Build history of the part. All positions in model axes, mm. Give positions to 0.01 mm unless a question says otherwise; leave off trailing zeros. Write each loop counter-clockwise with the first axis right and the second up, starting at its lowest first coordinate (ties: lowest second). Pieces come first, ordered by that corner, then holes. Notation, with made-up numbers: (52, 79.5) -> (70, 79.5) arc R37 ccw to (70, 115.5) -> close; hole circle Ø8 at (8, 16). An arc over 180 degrees is marked (long way). One line per question, with ' | ' between items. Start each with the question number.
(1) Pin check, flat tip, straight feed: P1, Ø5, axis at x = 30.75, y = -30.2, coming from the -Z side. Stop position of the tip, or through.
(2) Band-saw the part on B-B, the plane x = 0. Give the cut face in (y, z) (3 decimals).
(3) Drill centre lines: probe 1 along Y at (x, z) = (0, 19.5) (3 decimals); probe 2 along Y at (x, z) = (32, 5); probe 3 along X at (y, z) = (2, 11.75). Where is each one in solid material? Low to high. Write a range as from..to.
(4) Band-saw the part on A-A, the plane y = 0. Give the cut face in (x, z) (3 decimals).
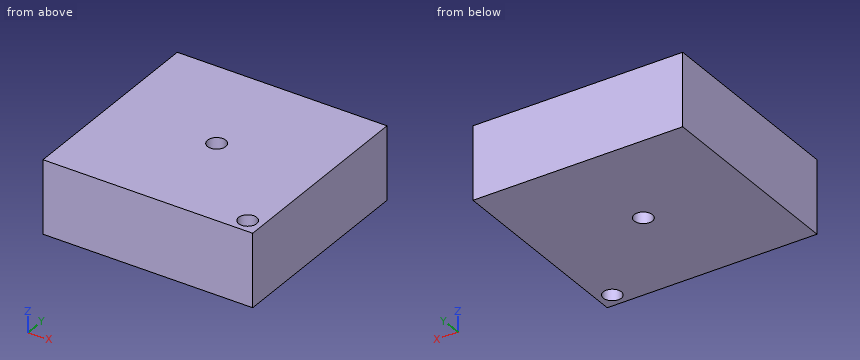
from build123d import *

# Parameters (mm, degrees)
F0_W     = 72.761286
F0_H     = 70.397198
F1_DEPTH = 25.4
F2_R     = 3.148558
F3_DEPTH = 25.4
F6_D     = 6.35


with BuildPart() as f1:
    # F0 (on Top) → F1 (new body)
    with BuildSketch(Plane.XY):
        with Locations((-0.571629, -0.002768)):
            Rectangle(F0_W, F0_H)
    extrude(amount=F1_DEPTH)


with BuildPart() as f3:
    # F2 (on Top) → F3 (new body)
    with BuildSketch(Plane.XY):
        with Locations((30.75167, -30.19508)):
            Circle(F2_R)
    extrude(amount=F3_DEPTH)


with BuildPart() as f1_1:
    add(f1.part)

    # F4: cut F3
    add(f3.part, mode=Mode.SUBTRACT)

    # F6 (through all)
    with Locations(Plane(origin=(0, 0, 0), x_dir=(1, 0, 0), z_dir=(0, 0, -1))):
        with Locations((0, 0)):
            Hole(F6_D / 2)


solid = f1_1.part
Results:
1) P1: passes through
2) outline: (-35.201, 0) -> (-3.175, 0) -> (-3.175, 25.4) -> (-35.201, 25.4) -> close; (3.175, 0) -> (35.196, 0) -> (35.196, 25.4) -> (3.175, 25.4) -> close
3) probe 1: y = -35.201..-3.175, 3.175..35.196 | probe 2: y = -35.2..-33.09, -27.3..35.2 | probe 3: x = -36.95..-2.47, 2.47..35.81
4) outline: (-36.952, 0) -> (-3.175, 0) -> (-3.175, 25.4) -> (-36.952, 25.4) -> close; (3.175, 0) -> (35.809, 0) -> (35.809, 25.4) -> (3.175, 25.4) -> close
